from build123d import *

# Parameters (mm, degrees)
SKETCH2_R           = 18.4
BOSS_EXTRUDE1_DEPTH = 24
SKETCH3_R           = 17
BOSS_EXTRUDE2_DEPTH = 46.1
CHAMFER1_SIZE       = 1
SKETCH6_R           = 6
BOSS_EXTRUDE5_DEPTH = 6
SKETCH7_R           = 3
BOSS_EXTRUDE6_DEPTH = 15
CUT_EXTRUDE1_DEPTH  = 12
CHAMFER2_SIZE       = 0.5
CIRPATTERN1_COUNT   = 6
SKETCH11_W          = 20
SKETCH11_H          = 2
BOSS_EXTRUDE7_DEPTH = 22


with BuildPart() as part:
    # Sketch2 → Boss-Extrude1 (new body)
    with BuildSketch(Plane.XY):
        Circle(SKETCH2_R)
    extrude(amount=BOSS_EXTRUDE1_DEPTH)

    # Sketch3 → Boss-Extrude2 (add)
    with BuildSketch(Plane(origin=(0, 0, 0), x_dir=(-1, 0, 0), z_dir=(0, 0, -1))):
        Circle(SKETCH3_R)
    extrude(amount=BOSS_EXTRUDE2_DEPTH)

    # Chamfer1
    chamfer1_edges = [part.edges().sort_by_distance(p)[0] for p in [
        (17, 0, -46.1),
    ]]
    chamfer(chamfer1_edges, length=CHAMFER1_SIZE)

    # Sketch6 → Boss-Extrude5 (add)
    with BuildSketch(Plane.XY.offset(24)):
        with Locations((0, 7.5)):
            Circle(SKETCH6_R)
    extrude(amount=BOSS_EXTRUDE5_DEPTH)

    # Sketch7 → Boss-Extrude6 (add)
    with BuildSketch(Plane.XY.offset(30)):
        with Locations((0, 7.5)):
            Circle(SKETCH7_R)
    extrude(amount=BOSS_EXTRUDE6_DEPTH)

    # Sketch8 → Cut-Extrude1 (cut)
    with BuildSketch(Plane.XY.offset(45)):
        Polygon((-81.196672921, 10), (-1.658312395, 10), (1.658312395, 10), (81.196672921, 10), (81.196672921, 169.076721051), (-81.196672921, 169.076721051), align=None)
    extrude(amount=-CUT_EXTRUDE1_DEPTH, mode=Mode.SUBTRACT)

    # Chamfer2
    chamfer2_edges = [part.edges().sort_by_distance(p)[0] for p in [
        (-1.418637165, 4.856617963, 45),
    ]]
    chamfer(chamfer2_edges, length=CHAMFER2_SIZE - 0.0001)  # a hair under: the kernel refuses the full size

    # Sketch10 → M3 Clearance Hole1 (revolve, cut)
    with BuildSketch(Plane(origin=(-15.5, 0, 24), x_dir=(0, -1, 0), z_dir=(1, 0, 0))):
        Polygon((0, 0), (0, 4.521463052), (1.7, 3.5), (1.7, 0), align=None)
    m3_clearance_hole1 = revolve(axis=Axis((-15.5, 0, 30.35), (0, 0, -1)), mode=Mode.SUBTRACT)

    # CirPattern1: M3 Clearance Hole1 ×6 about axis
    cirpattern1_axis = Axis((0, 0, 0), (0, 0, 1))
    for i in range(1, CIRPATTERN1_COUNT):
        add(m3_clearance_hole1.rotate(cirpattern1_axis, i * 360 / CIRPATTERN1_COUNT), mode=Mode.SUBTRACT)

    # Sketch11 → Boss-Extrude7 (add)
    with BuildSketch(Plane(origin=(0, 0, 0), x_dir=(1, 0, 0), z_dir=(0, 1, 0))):
        with Locations((0, 32.1)):
            Rectangle(SKETCH11_W, SKETCH11_H)
    extrude(amount=BOSS_EXTRUDE7_DEPTH)


solid = part.part
Read the model definition and answer for the solid it produces. Units are mm, in the model's axes. A direction names the side the tool comes from. Round coordinates to 2 decimals unless told otherwise and drop trailing zeros. Order: outer loops, then holes, each group sorted by start corner. A loop starts at its lowest first (then second) coordinate and runs counter-clockwise, first axis right, second up.
1) Straight lines are drawn through the part: L1, parallel to Z at x = -1, y = 17.5; L2, parallel to Y at x = -7, z = 22; L3, parallel to Z at x = 11.5, y = 7. For each, find the intervals that lie inside material, in ascending order.
2) The mould has two halves that part along X. Classify faces 4 (the face through (8.038, -13.359, 19.656)), 5 (the face through (-15.212, 0.064, 19.656)), 6 (the face through (-10, 18, -32)), 7 (the face through (0, 0, 24)): released by +X, released by -X, zero draft, split by the parting line, or undercut.
3) The part is cut by section B-B on z = 13. Write down the section's boundary in (x, y).
4) For faces 1 (the face through (0, 10, 39)), 2 (the face through (-3, 6, 30)), 3 (the face through (10, 18, -32)), determine the directions among +Z, -Z, +X, -X, +Y, -Y from which every point of the face is accessible in a straight line to the end or side of a thin tool.
5) The part is cut by section A-A on z = -22.5. Write down the section's boundary in (x, y), plus the area to 3 significant figures.
6) Flat-ended cylindrical pins translate along their axes: pin 1 (5.5 mm diameter, centred on x = -15.5, y = 0, fed in from +Z); pin 2 (5 mm diameter, centred on y = -13.5, z = 5, fed in from +X); pin 3 (1.5 mm diameter, centred on x = -4.5, z = -16.5, fed in from -Y). Find the tip coordinate at first contact, or state that the pin passes through.
Resolved:
1. L1: z = -33.1 to -31.1, 0 to 24
1. L2: y = -17.02 to -14.95, -11.9 to 11.9, 14.95 to 17.02
1. L3: z = -46.1 to 24
2. face 4: undercut
2. face 5: undercut
2. face 6: released by -X
2. face 7: zero draft
3. outline: circle Ø36.8 at (0, 0)
4. face 1: +Z, +X, -X, +Y
4. face 2: +Z
4. face 3: -Z, +X, +Y
5. outline: circle Ø34 at (0, 0)
5. area: 908 mm2
6. pin 1: stops at z = 24
6. pin 2: stops at x = 14.75
6. pin 3: stops at y = -16.58
